Here's how the part is built. I have some questions about the finished solid (model axes, mm). Coordinates: 2 decimals unless noted, no trailing zeros. Loops run counter-clockwise (first coordinate to the right, second up) from the corner with the lowest first, then second, coordinate; pieces in that order, holes last. Notation, with made-up numbers: (-5.5, 67.25) - (17.5, 67.25) arc R13 cw to (17.5, 85.25) - close; hole circle Ø6 at (-36, 31.5). An arc over 180 degrees is marked (long way). Use a Markdown table: item, result.
```python
from build123d import *

# Parameters (mm, degrees)
F1_DEPTH        = 12.7
F2_DEPTH        = 25.4
F2_COPIES_COUNT = 4
F3_R            = 19.04999
F5_R            = 50.8


# Not quite as in the source:
# - a fillet or chamfer is up to 0.001 mm smaller than in the source, because OpenCascade refuses the exact size
# - a feature of the source that left no trace in its solid (it failed there, or was rolled back) is left out
# - a pattern or mirror of a feature is missing from the dataset's text; its kind, count and spacing are read off the source's solid


with BuildPart() as f1:
    # F0 (on Top) → F1 (new body)
    with BuildSketch(Plane.XY):
        with BuildLine():
            Line((552.45, 95.25), (473.1069620075, 95.25))
            ThreePointArc((473.1069620075, 95.25), (480.2208761939, 47.8609451179), (482.6, 0))
            ThreePointArc((482.6, 0), (480.2208761939, -47.8609451179), (473.1069620075, -95.25))
            Line((473.1069620075, -95.25), (552.45, -95.25))
            Line((552.45, -95.25), (552.45, 95.25))
        make_face()
        with BuildLine():
            Line((-207.8109657838, 95.25), (-473.1069620075, 95.25))
            ThreePointArc((-473.1069620075, 95.25), (-480.2208762804, 47.8609442495), (-482.6, -1.7456e-06))
            ThreePointArc((-482.6, -1.7456e-06), (-480.2208761073, -47.8609459864), (-473.1069620075, -95.25))
            Line((-473.1069620075, -95.25), (-207.8109657838, -95.25))
            ThreePointArc((-207.8109657838, -95.25), (-228.6, 0), (-207.8109657838, 95.25))
        make_face()
        with BuildLine():
            Line((473.1069620075, 95.25), (207.8109657838, 95.25))
            ThreePointArc((207.8109657838, 95.25), (223.3422785527, 48.7461445748), (228.6, 0))
            ThreePointArc((228.6, 0), (223.3422785527, -48.7461445748), (207.8109657838, -95.25))
            Line((207.8109657838, -95.25), (473.1069620075, -95.25))
            ThreePointArc((473.1069620075, -95.25), (480.2208761939, -47.8609451179), (482.6, 0))
            ThreePointArc((482.6, 0), (480.2208761939, 47.8609451179), (473.1069620075, 95.25))
        make_face()
        with BuildLine():
            ThreePointArc((-458.9465033909, 149.2342689375), (-466.8077665522, 122.4470052167), (-473.1069620075, 95.25))
            Line((-473.1069620075, 95.25), (-207.8109657838, 95.25))
            ThreePointArc((-207.8109657838, 95.25), (-161.6446101792, 161.6446101792), (-95.25, 207.8109657838))
            Line((-95.25, 207.8109657838), (-95.25, 473.1069620075))
            ThreePointArc((-95.25, 473.1069620075), (-122.4470052167, 466.8077665522), (-149.2342689375, 458.9465033909))
            ThreePointArc((-149.2342689375, 458.9465033909), (-341.2497326006, 341.2497326006), (-458.9465033909, 149.2342689375))
        make_face()
        with BuildLine():
            Line((-95.25, 473.1069620075), (-95.25, 207.8109657838))
            ThreePointArc((-95.25, 207.8109657838), (0, 228.6), (95.25, 207.8109657838))
            Line((95.25, 207.8109657838), (95.25, 473.1069620075))
            ThreePointArc((95.25, 473.1069620075), (0, 482.6), (-95.25, 473.1069620075))
        make_face()
        with BuildLine():
            Line((95.25, 473.1069620075), (95.25, 207.8109657838))
            ThreePointArc((95.25, 207.8109657838), (161.6446101792, 161.6446101792), (207.8109657838, 95.25))
            Line((207.8109657838, 95.25), (473.1069620075, 95.25))
            ThreePointArc((473.1069620075, 95.25), (466.8077665522, 122.4470052167), (458.9465033909, 149.2342689375))
            ThreePointArc((458.9465033909, 149.2342689375), (341.2497326006, 341.2497326006), (149.2342689375, 458.9465033909))
            ThreePointArc((149.2342689375, 458.9465033909), (122.4470052167, 466.8077665522), (95.25, 473.1069620075))
        make_face()
        with BuildLine():
            Line((-95.25, 552.45), (-95.25, 473.1069620075))
            ThreePointArc((-95.25, 473.1069620075), (0, 482.6), (95.25, 473.1069620075))
            Line((95.25, 473.1069620075), (95.25, 552.45))
            Line((95.25, 552.45), (-95.25, 552.45))
        make_face()
        with BuildLine():
            ThreePointArc((207.8109657838, -95.25), (161.6446101792, -161.6446101792), (95.25, -207.8109657838))
            Line((95.25, -207.8109657838), (95.25, -473.1069620075))
            ThreePointArc((95.25, -473.1069620075), (122.4470052167, -466.8077665522), (149.2342689375, -458.9465033909))
            ThreePointArc((149.2342689375, -458.9465033909), (341.2497326006, -341.2497326006), (458.9465033909, -149.2342689375))
            ThreePointArc((458.9465033909, -149.2342689375), (466.8077665522, -122.4470052167), (473.1069620075, -95.25))
            Line((473.1069620075, -95.25), (207.8109657838, -95.25))
        make_face()
        with BuildLine():
            ThreePointArc((95.25, -207.8109657838), (0, -228.6), (-95.25, -207.8109657838))
            Line((-95.25, -207.8109657838), (-95.25, -473.1069620075))
            ThreePointArc((-95.25, -473.1069620075), (0, -482.6), (95.25, -473.1069620075))
            Line((95.25, -473.1069620075), (95.25, -207.8109657838))
        make_face()
        with BuildLine():
            Line((-207.8109657838, -95.25), (-473.1069620075, -95.25))
            ThreePointArc((-473.1069620075, -95.25), (-466.8077665522, -122.4470052167), (-458.9465033909, -149.2342689375))
            ThreePointArc((-458.9465033909, -149.2342689375), (-341.2497326006, -341.2497326006), (-149.2342689375, -458.9465033909))
            ThreePointArc((-149.2342689375, -458.9465033909), (-122.4470052167, -466.8077665522), (-95.25, -473.1069620075))
            Line((-95.25, -473.1069620075), (-95.25, -207.8109657838))
            ThreePointArc((-95.25, -207.8109657838), (-161.6446101792, -161.6446101792), (-207.8109657838, -95.25))
        make_face()
        with BuildLine():
            ThreePointArc((95.25, -473.1069620075), (0, -482.6), (-95.25, -473.1069620075))
            Line((-95.25, -473.1069620075), (-95.25, -552.45))
            Line((-95.25, -552.45), (95.25, -552.45))
            Line((95.25, -552.45), (95.25, -473.1069620075))
        make_face()
        with BuildLine():
            Line((-473.1069620075, 95.25), (-552.45, 95.25))
            Line((-552.45, 95.25), (-552.45, -95.25))
            Line((-552.45, -95.25), (-473.1069620075, -95.25))
            ThreePointArc((-473.1069620075, -95.25), (-480.2208761073, -47.8609459864), (-482.6, -1.7456e-06))
            ThreePointArc((-482.6, -1.7456e-06), (-480.2208762804, 47.8609442495), (-473.1069620075, 95.25))
        make_face()
        Polygon((-482.6, 82.55), (-482.6, -1.7456e-06), (-482.6, -82.55), (-520.7, -82.55), (-520.7, 82.55), align=None, mode=Mode.SUBTRACT)
        Polygon((-482.6, -82.55), (-482.6, -1.7456e-06), (-482.6, 82.55), (-520.7, 82.55), (-520.7, -82.55), align=None)
        with BuildLine():
            Line((-458.9465033909, 149.2342689375), (-552.45, 95.25))
            Line((-552.45, 95.25), (-473.1069620075, 95.25))
            ThreePointArc((-473.1069620075, 95.25), (-466.8077665522, 122.4470052167), (-458.9465033909, 149.2342689375))
        make_face()
        with BuildLine():
            Line((-473.1069620075, -95.25), (-552.45, -95.25))
            Line((-552.45, -95.25), (-458.9465033909, -149.2342689375))
            ThreePointArc((-458.9465033909, -149.2342689375), (-466.8077665522, -122.4470052167), (-473.1069620075, -95.25))
        make_face()
        with BuildLine():
            Line((-95.25, 552.45), (-149.2342689375, 458.9465033909))
            ThreePointArc((-149.2342689375, 458.9465033909), (-122.4470052167, 466.8077665522), (-95.25, 473.1069620075))
            Line((-95.25, 473.1069620075), (-95.25, 552.45))
        make_face()
        with BuildLine():
            Line((95.25, 552.45), (95.25, 473.1069620075))
            ThreePointArc((95.25, 473.1069620075), (122.4470052167, 466.8077665522), (149.2342689375, 458.9465033909))
            Line((149.2342689375, 458.9465033909), (95.25, 552.45))
        make_face()
        with BuildLine():
            ThreePointArc((458.9465033909, 149.2342689375), (466.8077665522, 122.4470052167), (473.1069620075, 95.25))
            Line((473.1069620075, 95.25), (552.45, 95.25))
            Line((552.45, 95.25), (458.9465033909, 149.2342689375))
        make_face()
        with BuildLine():
            Line((552.45, -95.25), (473.1069620075, -95.25))
            ThreePointArc((473.1069620075, -95.25), (466.8077665522, -122.4470052167), (458.9465033909, -149.2342689375))
            Line((458.9465033909, -149.2342689375), (552.45, -95.25))
        make_face()
        with BuildLine():
            ThreePointArc((149.2342689375, -458.9465033909), (122.4470052167, -466.8077665522), (95.25, -473.1069620075))
            Line((95.25, -473.1069620075), (95.25, -552.45))
            Line((95.25, -552.45), (149.2342689375, -458.9465033909))
        make_face()
        with BuildLine():
            ThreePointArc((-95.25, -473.1069620075), (-122.4470052167, -466.8077665522), (-149.2342689375, -458.9465033909))
            Line((-149.2342689375, -458.9465033909), (-95.25, -552.45))
            Line((-95.25, -552.45), (-95.25, -473.1069620075))
        make_face()
    extrude(amount=-F1_DEPTH)

    # F0 (on Top) → F2 (cut)
    with BuildSketch(Plane.XY):
        Polygon((-482.6, -82.55), (-482.6, -1.7456e-06), (-482.6, 82.55), (-520.7, 82.55), (-520.7, -82.55), align=None)
    f2 = extrude(amount=-F2_DEPTH, mode=Mode.SUBTRACT)

    # F2_copies: F2 ×4 about axis
    f2_copies_axis = Axis((0, 0, 0), (0, 0, 1))
    for i in range(1, F2_COPIES_COUNT):
        add(f2.rotate(f2_copies_axis, i * 360 / F2_COPIES_COUNT), mode=Mode.SUBTRACT)

    # F3 (radius 19.05 in the source; OpenCascade refuses exactly that, so slightly less here)
    f3_edges = [f1.edges().sort_by_distance(p)[0] for p in [
        (-520.7, -82.55, -6.35),
        (-482.6, -82.55, -6.35),
        (-520.7, 82.55, -6.35),
        (-482.6, 82.55, -6.35),
        (-82.55, -520.7, -6.35),
        (-82.55, -482.6, -6.35),
        (82.55, -482.6, -6.35),
        (82.55, -520.7, -6.35),
        (520.7, -82.55, -6.35),
        (482.6, -82.55, -6.35),
        (482.6, 82.55, -6.35),
        (520.7, 82.55, -6.35),
        (82.55, 520.7, -6.35),
        (82.55, 482.6, -6.35),
        (-82.55, 520.7, -6.35),
        (-82.55, 482.6, -6.35),
    ]]
    fillet(f3_edges, radius=F3_R)

    # F5
    f5_edges = [f1.edges().sort_by_distance(p)[0] for p in [
        (-149.234269, -458.946503, -6.35),
        (-95.25, -552.45, -6.35),
        (95.25, -552.45, -6.35),
        (149.234269, -458.946503, -6.35),
        (458.946503, -149.234269, -6.35),
        (552.45, -95.25, -6.35),
        (552.45, 95.25, -6.35),
        (458.946503, 149.234269, -6.35),
        (149.234269, 458.946503, -6.35),
        (95.25, 552.45, -6.35),
        (-95.25, 552.45, -6.35),
        (-149.234269, 458.946503, -6.35),
        (-458.946503, 149.234269, -6.35),
        (-552.45, 95.25, -6.35),
        (-552.45, -95.25, -6.35),
        (-458.946503, -149.234269, -6.35),
    ]]
    fillet(f5_edges, radius=F5_R)


solid = f1.part
```
Q1. I want a section at D-D, the plane x = 305. Write out the boundary of the cut face in (y, z).
Check values:
| item | result |
|---|---|
| outline | (-374, -12.7) - (374, -12.7) - (374, 0) - (-374, 0) - close |
Q2. I want a section at C-C, the plane y = -256. Write out the boundary of the cut face in (x, z), then the cut area to 3 significant figures.
Check values:
| item | result |
|---|---|
| outline | (-409.1, -12.7) - (409.1, -12.7) - (409.1, 0) - (-409.1, 0) - close |
| area | 10,400 mm^2 |
Q3. Will these pins go through, and if not, where does the flat tip stop? P1, Ø3, axis at x = -290, z = -7.5, coming from the +Y side; P2, Ø4, axis at y = 174.5, z = -4, coming from the -X side.
Check values:
| item | result |
|---|---|
| P1 | y = 386.87 |
| P2 | x = -450.72 |
Q4. I want a section at A-A, the plane x = -12.5. Write out the boundary of the cut face in (y, z).
Check values:
| item | result |
|---|---|
| outline | (-552.45, -12.7) - (-520.7, -12.7) - (-520.7, 0) - (-552.45, 0) - close; (-482.6, -12.7) - (-228.26, -12.7) - (-228.26, 0) - (-482.6, 0) - close; (228.26, -12.7) - (482.6, -12.7) - (482.6, 0) - (228.26, 0) - close; (520.7, -12.7) - (552.45, -12.7) - (552.45, 0) - (520.7, 0) - close |
Q5. Please list where these lines run through material, in increasing order: L1, parallel to Y at x = 69, z = -4.5; L2, parallel to Y at x = 39, z = -3.5; L3, parallel to Y at x = 92.5, z = -2.25. Write a range as from..to.
Check values:
| item | result |
|---|---|
| L1 | -552.36..-519.89, -483.41..-217.94, 217.94..483.41, 519.89..552.36 |
| L2 | -552.45..-520.7, -482.6..-225.25, 225.25..482.6, 520.7..552.45 |
| L3 | -544.94..-209.05, 209.05..544.94 |
Q6. I want a section at B-B, the plane z = -10.75. Give the number of separate pieces and of enclosed holes in the cut face, then the cut area to 3 significant figures.
Check values:
| item | result |
|---|---|
| separate pieces | 1 |
| enclosed holes | 5 |
| area | 615,000 mm^2 |
